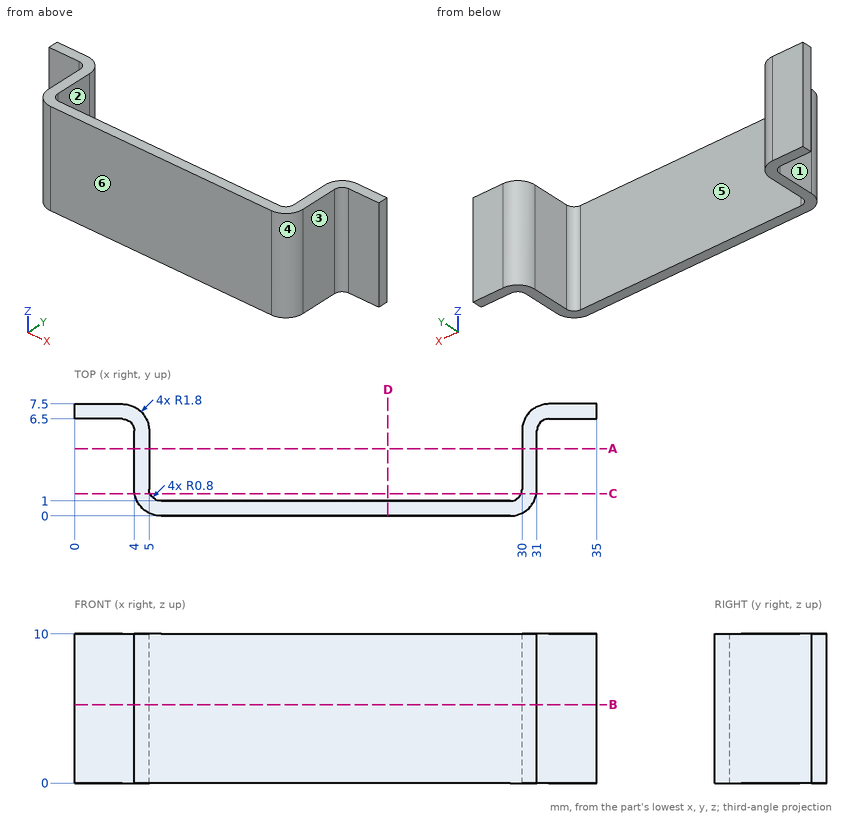
Geometry: see drawing. Coordinates: mm, zero at the bounding-box minimum. A direction names the side the tool comes from. Give positions to 0.01 mm unless a question says otherwise; leave off trailing zeros. Order: outer loops, then holes, each group sorted by start corner. A loop starts at its lowest first (then second) coordinate and runs counter-clockwise, first axis right, second up. Notation, with made-up numbers: (19.5, 68.5) -> (35.5, 68.5) arc R28 ccw to (35.5, 92.5) -> close; hole circle Ø4 at (-36.5, 24). An arc over 180 degrees is marked (long way). Write item = value, one per line.
Q1. Cut plane B-B, the plane z = 5.25. Output: boundary loops of the cut face in (x, y), and give its area (3 significant figures).
Data:
outline = (0, 6.5) -> (3.2, 6.5) arc R0.8 cw to (4, 5.7) -> (4, 1.8) arc R1.8 ccw to (5.8, 0) -> (29.2, 0) arc R1.8 ccw to (31, 1.8) -> (31, 5.7) arc R0.8 cw to (31.8, 6.5) -> (35, 6.5) -> (35, 7.5) -> (31.8, 7.5) arc R1.8 ccw to (30, 5.7) -> (30, 1.8) arc R0.8 cw to (29.2, 1) -> (5.8, 1) arc R0.8 cw to (5, 1.8) -> (5, 5.7) arc R1.8 ccw to (3.2, 7.5) -> (0, 7.5) -> close
area = 45.8 mm^2
Q2. Cut plane C-C, the plane y = 1.5. Output: boundary loops of the cut face in (x, z).
Data:
outline = (4.03, 0) -> (5.06, 0) -> (5.06, 10) -> (4.03, 10) -> close; (29.94, 0) -> (30.97, 0) -> (30.97, 10) -> (29.94, 10) -> close
Q3. Set-up query: the marked faces 1, 2 and 3. Return all of +Z, -Z, +X, -X, +Y, -Y with unobstructed straight access to the full face (end or side cutting, diameter ignored); none if empty.
Data:
face_1 = +Z, -Z, -X, -Y
face_2 = +Z, -Z, +Y
face_3 = +Z, -Z, +X, -Y
Q4. Pull-direction query (X, two-part tool) for the marked faces 4, 5 and 6; classes: released by +X, released by -X, zero draft, split by the parting line, or undercut.
Data:
face_4 = released by +X
face_5 = undercut
face_6 = zero draft
Q5. Pin query (flat end, axial travel): pin 1 (3 mm diameter, centred on y = 4.5, z = 7.5, fed in from -X); pin 2 (1.5 mm diameter, centred on y = 5, z = 8, fed in from +X); pin 3 (4.5 mm diameter, centred on y = 3.5, z = 7, fed in from -X). Return the tip coordinate at first contact, or that it passes through.
Data:
pin_1 = 3.94
pin_2 = 31
pin_3 = 4
Q6. Cut plane A-A, the plane y = 4.5. Output: boundary loops of the cut face in (x, z).
Data:
outline = (4, 0) -> (5, 0) -> (5, 10) -> (4, 10) -> close; (30, 0) -> (31, 0) -> (31, 10) -> (30, 10) -> close
Q7. Cut plane D-D, the plane x = 21. Output: boundary loops of the cut face in (y, z), and give its area (3 significant figures).
Data:
outline = (0, 0) -> (1, 0) -> (1, 10) -> (0, 10) -> close
area = 10.0 mm^2
Q8. Material intervals for line 1 (X direction, y = 4, z = 5.75); line 2 (Y direction, x = 2.5, z = 1); line 3 (Y direction, x = 19.5, z = 0.75), sorted ascending. Write a range as from..to.
Data:
line_1 = 4..5, 30..31
line_2 = 6.5..7.5
line_3 = 0..1
